Here's how the part is built. I have some questions about the finished solid (model axes, mm). Give positions to 0.01 mm unless a question says otherwise; leave off trailing zeros. Loops run counter-clockwise (first coordinate to the right, second up) from the corner with the lowest first, then second, coordinate; pieces in that order, holes last. Notation, with made-up numbers: (41.5, 78.25) - (57.5, 78.25) arc R30 cw to (57.5, 100.25) - close; hole circle Ø1 at (-0.75, 75). An arc over 180 degrees is marked (long way). Return JSON: item names as keys, results as strings. Group by question number.
(1) If we section it at B-B (x = 0): Please give me the cut outline in (y, z) (1 decimal).
(2) I need wall thicknesses on probe 1 along Z at (x, y) = (1, 2.5); probe 2 along X at (y, z) = (1.6, 0); probe 3 along X at (y, z) = (2.8, 5). Which ranges of each line are inside material? Lowest first, please. Write a range as [from, to].
(3) For P1, Ø3.5, axis at x = -16.84, z = 9.49, coming from the +Y side; P2, Ø1.5, axis at y = 1, z = -29, coming from the +X side; P3, Ø1.5, axis at y = 1.5, z = 12, coming from the +X side, each with a flat end and sliding along its axis, tell me the tip position at first contact or that it passes through.
(4) If we section it at D-D (z = -19.05): Please give me the cut outline in (x, y) (3 decimals).
(5) If we section it at A-A (z = 0): Please give me the cut outline in (x, y) (1 decimal).
(6) If we section it at C-C (y = 1.9): State how many separate pieces and enclosed holes the cut face has, then the cut area to 3 significant figures.
(7) If we mould it in two halves opening along X, with no side actions, what happens to faces 1 (the cylindrical face through (11.487, 1.565, 36.478)), 2 (the cylindrical face through (0.628, 1.565, 14.274)), 3 (the flat face through (1, 0, 16))? For each: released by +X, released by -X, zero draft, split by the parting line, or undercut.
```python
from build123d import *

# Parameters (mm, degrees)
SKETCH1_R           = 38.243875115
SKETCH1_R_2         = 12.860433797
SKETCH1_R_3         = 2.952880618
SKETCH1_R_4         = 2.979621757
SKETCH1_R_5         = 2.909102137
BOSS_EXTRUDE1_DEPTH = 3.175
SKETCH2_R           = 14.2875
CUT_EXTRUDE1_DEPTH  = 3.175


with BuildPart() as part:
    # Sketch1 → Boss-Extrude1 (new body)
    with BuildSketch(Plane(origin=(0, 0, 0), x_dir=(1, 0, 0), z_dir=(0, 1, 0))):
        with Locations(Location((0, 0, 0), (0, 0, 270))):
            Circle(SKETCH1_R)
        with Locations(Location((0, 0, 0), (0, 0, 270))):
            Circle(SKETCH1_R_2, mode=Mode.SUBTRACT)
        with Locations(Location((-16.841170726, -9.494245367, 0), (0, 0, 270))):
            Circle(SKETCH1_R_3, mode=Mode.SUBTRACT)
        with Locations(Location((16.444515355, -9.494245367, 0), (0, 0, 270))):
            Circle(SKETCH1_R_4, mode=Mode.SUBTRACT)
        with Locations(Location((0, 19.05, 0), (0, 0, 270))):
            Circle(SKETCH1_R_5, mode=Mode.SUBTRACT)
    extrude(amount=BOSS_EXTRUDE1_DEPTH)

    # Sketch2 → Cut-Extrude1 (cut)
    with BuildSketch(Plane.XZ):
        with Locations(Location((0, 0, 0), (0, 0, 270))):
            Circle(SKETCH2_R)
    extrude(amount=-CUT_EXTRUDE1_DEPTH, mode=Mode.SUBTRACT)


solid = part.part
```
Values:
{
 "1": {"outline": "(0, -38.2) - (3.2, -38.2) - (3.2, -22) - (0, -22) - close; (0, -16.1) - (3.2, -16.1) - (3.2, -14.3) - (0, -14.3) - close; (0, 14.3) - (3.2, 14.3) - (3.2, 38.2) - (0, 38.2) - close"},
 "2": {"probe 1": "[-38.23, -21.78], [-16.32, -14.25], [14.25, 38.23]", "probe 2": "[-38.24, -14.29], [14.29, 38.24]", "probe 3": "[-37.92, -13.38], [13.38, 37.92]"},
 "3": {"P1": "through", "P2": "x = 25.78", "P3": "x = 36.55"},
 "4": {"outline": "(-33.162, 0) - (-2.909, 0) - (-2.909, 3.175) - (-33.162, 3.175) - close; (2.909, 0) - (33.162, 0) - (33.162, 3.175) - (2.909, 3.175) - close"},
 "5": {"outline": "(-38.2, 0) - (-14.3, 0) - (-14.3, 3.2) - (-38.2, 3.2) - close; (14.3, 0) - (38.2, 0) - (38.2, 3.2) - (14.3, 3.2) - close"},
 "6": {"separate pieces": "1", "enclosed holes": "4", "area": "3,870 mm2"},
 "7": {"face 1": "split by the parting line", "face 2": "undercut", "face 3": "zero draft"}
}
